Read the model definition and answer for the solid it produces. Units are mm, in the model's axes. Face numbers are marked on the shaded views. Coordinates: 2 decimals unless noted, no trailing zeros. Write each loop counter-clockwise with the first axis right and the second up, starting at its lowest first coordinate (ties: lowest second). Pieces come first, ordered by that corner, then holes. Notation, with made-up numbers: M 82.5,79 L 137.5,79 A33 ccw 137.5,109 Z; hole C -38.5,30.25 d6. An arc over 180 degrees is marked long. Use a Markdown table: item, result. Add a question column.
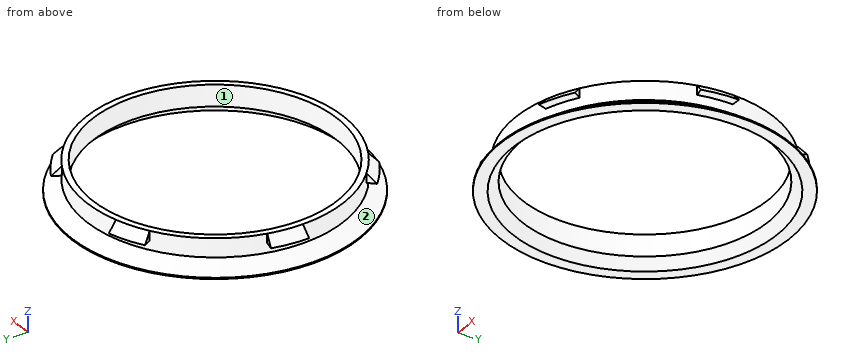
from build123d import *

# Parameters (mm, degrees)
REVOLUTION001_ANGLE = -15
POLARPATTERN_COUNT  = 6
CHAMFER_SIZE        = 3


with BuildPart() as part:
    # Sketch → Revolution (revolve)
    with BuildSketch(Plane.XZ):
        Polygon((-42, 10), (-40, 10), (-40, 0), (-47, 0), (-47, 0.4), (-42, 3.901038), align=None)
    revolve(axis=Axis((0, 0, 0), (0, 0, 1)))

    # Sketch001 → Revolution001 (revolve)
    with BuildSketch(Plane.XZ):
        Polygon((-45, 7), (-42, 7), (-42, 10), align=None)
    revolution001 = revolve(axis=Axis((0, 0, 0), (0, 0, 1)), revolution_arc=REVOLUTION001_ANGLE)

    # PolarPattern: Revolution001 ×6 about axis
    polarpattern_axis = Axis((0, 0, 0), (0, 0, 1))
    for i in range(1, POLARPATTERN_COUNT):
        add(revolution001.rotate(polarpattern_axis, i * 360 / POLARPATTERN_COUNT))

    # Chamfer
    chamfer_edges = [part.edges().sort_by_distance(p)[0] for p in [
        (40, 0, 0),
    ]]
    chamfer(chamfer_edges, length=CHAMFER_SIZE)


solid = part.part
Item 1: Determine the mould class of the marked faces 1 and 2 for opening direction Y: pulls with the +Y half, pulls with the -Y half, needs draft (parallel to the pull), parting line crosses it, or undercut.
Item 2: Find section B-B on z = 5. Give the vertices of the cut face in (x, y).
Item 3: Consider probe 1 along X at (y, z) = (0, 5); probe 2 along Y at (x, z) = (3.5, 9.25). Determine where each line is inside the solid, lowest interval first.
Item 4: Each of these flat-tipped pins is pushed along its axis until it touches: pin 1 (5 mm diameter, centred on x = -5, z = 2.5, fed in from -Y); pin 2 (2 mm diameter, centred on x = -14, z = 6, fed in from -Y); pin 3 (4 mm diameter, centred on x = 31, y = -20, fed in from +Z); pin 4 (1.5 mm diameter, centred on x = -30.5, z = 5.5, fed in from +Y). Where does it stop, or does it pass through?
Item 5: Find section A-A on x = 0. Give the vertices of the cut face in (y, z).
Geometry says:
| question | item | result |
|---|---|---|
| 1 | face 1 | undercut |
| 1 | face 2 | parting line crosses it |
| 2 | outline | C 0,0 d84; hole C 0,0 d80 |
| 3 | probe 1 | x = -42 to -40, 40 to 42 |
| 3 | probe 2 | y = -41.85 to -39.85, 39.85 to 41.85 |
| 4 | pin 1 | stops at y = -46.86 |
| 4 | pin 2 | stops at y = -39.94 |
| 4 | pin 3 | passes through |
| 4 | pin 4 | stops at y = 29.65 |
| 5 | outline | M -47,0 L -43,0 L -40,3 L -40,10 L -42,10 L -42,3.9 L -47,0.4 Z; M 40,3 L 43,0 L 47,0 L 47,0.4 L 42,3.9 L 42,10 L 40,10 Z |
